For this review, take the finished solid that the model builds, in its own axes (mm). A direction names the side the tool comes from. Round coordinates to 2 decimals unless told otherwise and drop trailing zeros. Write each loop counter-clockwise with the first axis right and the second up, starting at its lowest first coordinate (ties: lowest second). Pieces come first, ordered by that corner, then holes. Notation, with made-up numbers: M 16,53.25 L 54,53.25 A24 ccw 54,66.25 Z; hole C 65,84.25 d9. An arc over 180 degrees is marked long. Answer in a Markdown table with one row per item.
```python
from build123d import *

# Parameters (mm, degrees)
BOSS_EXTRUDE1_DEPTH = 190.5
BOSS_EXTRUDE2_DEPTH = 50.8
SKETCH3_R           = 3.175
BOSS_EXTRUDE3_DEPTH = 50.8
SKETCH4_W           = 15.875
SKETCH4_H           = 9.525
CUT_EXTRUDE1_DEPTH  = 31.1625
SKETCH5_R           = 3.175
CUT_EXTRUDE2_DEPTH  = 61.325


with BuildPart() as part:
    # Sketch1 → Boss-Extrude1 (new body, symmetric)
    with BuildSketch(Plane.XY):
        with BuildLine():
            Line((-19.05, -12.7), (19.05, -12.7))
            ThreePointArc((19.05, -12.7), (23.540128061, -10.840128061), (25.4, -6.35))
            Line((25.4, -6.35), (25.4, 6.35))
            ThreePointArc((25.4, 6.35), (23.540128061, 10.840128061), (19.05, 12.7))
            Line((19.05, 12.7), (-19.05, 12.7))
            ThreePointArc((-19.05, 12.7), (-23.540128061, 10.840128061), (-25.4, 6.35))
            Line((-25.4, 6.35), (-25.4, -6.35))
            ThreePointArc((-25.4, -6.35), (-23.540128061, -10.840128061), (-19.05, -12.7))
        make_face()
        with BuildLine():
            Line((-19.05, 11.049), (19.05, 11.049))
            ThreePointArc((19.05, 11.049), (22.372694765, 9.672694765), (23.749, 6.35))
            Line((23.749, 6.35), (23.749, -6.35))
            ThreePointArc((23.749, -6.35), (22.372694765, -9.672694765), (19.05, -11.049))
            Line((19.05, -11.049), (-19.05, -11.049))
            ThreePointArc((-19.05, -11.049), (-22.372694765, -9.672694765), (-23.749, -6.35))
            Line((-23.749, -6.35), (-23.749, 6.35))
            ThreePointArc((-23.749, 6.35), (-22.372694765, 9.672694765), (-19.05, 11.049))
        make_face(mode=Mode.SUBTRACT)
    extrude(amount=BOSS_EXTRUDE1_DEPTH, both=True)

    # Sketch2 → Boss-Extrude2 (add, through all)
    with BuildSketch(Plane(origin=(25.4, 0, 0), x_dir=(0, 0, -1), z_dir=(1, 0, 0))):
        with BuildLine():
            Line((177.8, -12.7), (177.8, -17.4625))
            Line((177.8, -17.4625), (195.2625, -17.4625))
            ThreePointArc((195.2625, -17.4625), (198.630096045, -9.332403955), (190.5, -12.7))
            Line((190.5, -12.7), (177.8, -12.7))
        make_face()
    boss_extrude2 = extrude(amount=-BOSS_EXTRUDE2_DEPTH)

    # Mirror1: Boss-Extrude2 across plane
    add(boss_extrude2.mirror(Plane.XY))

    # Sketch3 → Boss-Extrude3 (add, symmetric)
    with BuildSketch(Plane(origin=(0, 0, 0), x_dir=(0, 0, -1), z_dir=(1, 0, 0))):
        with Locations((195.2625, -12.7)):
            Circle(SKETCH3_R)
    extrude(amount=BOSS_EXTRUDE3_DEPTH, both=True)

    # Sketch4 → Cut-Extrude1 (cut, through all)
    with BuildSketch(Plane.XZ.offset(17.4625)):
        with Locations((-17.4625, 195.2625)):
            Rectangle(SKETCH4_W, SKETCH4_H)
        with Locations((17.4625, 195.2625)):
            Rectangle(SKETCH4_W, SKETCH4_H)
    extrude(amount=-CUT_EXTRUDE1_DEPTH, mode=Mode.SUBTRACT)

    # Sketch5 → Cut-Extrude2 (cut, through all)
    with BuildSketch(Plane(origin=(9.525, 0, 0), x_dir=(0, 0, -1), z_dir=(1, 0, 0))):
        with Locations((-195.2625, -12.7)):
            Circle(SKETCH5_R)
    extrude(amount=-CUT_EXTRUDE2_DEPTH, mode=Mode.SUBTRACT)


solid = part.part
```
Q1. Take a section at A-A (y = -1). State the section outline as (x, z) points, then the cut area to 3 significant figures.
Found:
| item | result |
|---|---|
| outline | M -25.4,-190.5 L -23.75,-190.5 L -23.75,190.5 L -25.4,190.5 Z; M 23.75,-190.5 L 25.4,-190.5 L 25.4,190.5 L 23.75,190.5 Z |
| area | 1,260 mm² |
Q2. Insertion check: P1, Ø10, axis at x = 35.5, y = -2.5, coming from the -Z side; P2, Ø7, axis at x = 24, z = 184, coming from the +Y side; P3, Ø11.5, axis at x = 6.5, z = 6, coming from the -Y side; P4, Ø3, axis at y = -14.5, z = 195.5, coming from the -X side (3 decimals). Each pin has a flat end and moves straight along its axis. Give the tip position at first contact, or say it passes through.
Found:
| item | result |
|---|---|
| P1 | through |
| P2 | y = 12.53 |
| P3 | y = -12.7 |
| P4 | x = -9.525 |
Q3. For probe 1 along X at (y, z) = (0.5, -56); probe 2 along Y at (x, z) = (-11.5, 180.5); probe 3 along Y at (x, z) = (0, -121.5), list the stretches that pass through material, from the lowest coordinate up.
Found:
| item | result |
|---|---|
| probe 1 | -25.4 to -23.75, 23.75 to 25.4 |
| probe 2 | -17.46 to -11.05, 11.05 to 12.7 |
| probe 3 | -12.7 to -11.05, 11.05 to 12.7 |
Q4. Take a section at B-B (z = -66). State the section outline as (x, y) points, then the cut area to 3 significant figures.
Found:
| item | result |
|---|---|
| outline | M -25.4,-6.35 A6.35 ccw -19.05,-12.7 L 19.05,-12.7 A6.35 ccw 25.4,-6.35 L 25.4,6.35 A6.35 ccw 19.05,12.7 L -19.05,12.7 A6.35 ccw -25.4,6.35 Z; hole M -23.75,-6.35 A4.7 ccw -19.05,-11.05 L 19.05,-11.05 A4.7 ccw 23.75,-6.35 L 23.75,6.35 A4.7 ccw 19.05,11.05 L -19.05,11.05 A4.7 ccw -23.75,6.35 Z |
| area | 225 mm² |
Q5. Machinability: for faces 5 (the face through (-0.1, 11.3, -190.5)), 6 (the face through (-37.9, -13.9, -198.2)), 7 (the face through (-9.525, -16, 194)), which of the approach directions +Z, -Z, +X, -X, +Y, -Y give a long, thin tool a straight path to every point of the face, cutting with its end or side? Answer none if there is none.
Found:
| item | result |
|---|---|
| face 5 | none |
| face 6 | -X |
| face 7 | +Z, -X, +Y, -Y |
Q6. Mouldability with a two-part tool opening along X and no side actions: class faces 1 (the face through (-23.49, 10.89, 2.67)), 2 (the face through (0, 11.049, 3)), 3 (the face through (0, -12.7, 2)), 4 (the face through (23.749, 0, 3)) as +X half, -X half, draft (parallel to the pull), parting line (faces both ways), or undercut.
Found:
| item | result |
|---|---|
| face 1 | -X half |
| face 2 | undercut |
| face 3 | draft |
| face 4 | undercut |
Q7. Take a section at C-C (x = 14.5). State the section outline as (y, z) points (1 decimal), then the cut area to 3 significant figures.
Found:
| item | result |
|---|---|
| outline | M -17.5,-195.3 A4.8 ccw long -12.7,-190.5 L -11,-190.5 L -11,190.5 L -17.5,190.5 L -17.5,177.8 L -12.7,177.8 L -12.7,-177.8 L -17.5,-177.8 Z; M 11,-190.5 L 12.7,-190.5 L 12.7,190.5 L 11,190.5 Z |
| area | 1,460 mm² |
